from build123d import *

# Parameters (mm, degrees)
F0_W        = 127
F0_H        = 127
F1_DEPTH    = 19.05
F2_T1_DEPTH = 257.6414957887
F2_T3_DEPTH = 257.6414957887
F3_T        = -2.54
F4_W        = 63.5
F4_H        = 63.5
F5_DEPTH    = 25.4


# Not quite as in the source:
# - a fillet or chamfer that OpenCascade refuses, or shapes differently, is made with other operations: its cross-section is extruded or revolved along the edge and cut away or added


with BuildPart() as f1:
    # F0 (on Front) → F1 (new body)
    with BuildSketch(Plane.XZ):
        with Locations((-51.5997745097, 45.6864875067)):
            Rectangle(F0_W, F0_H)
    extrude(amount=F1_DEPTH)

    # F2: chamfer of 25.4 on 4 edges, made by hand

    # F2_s2 → F2_t1 (cut)
    with BuildSketch(Plane.XY.offset(-83.1342603876)):
        Polygon((11.9002254903, 6.35), (-13.4997745097, -19.05), (11.9002254903, -19.05), align=None)
        Polygon((-115.0997745097, 6.35), (-89.6997745097, -19.05), (-115.0997745097, -19.05), align=None)
    extrude(amount=F2_T1_DEPTH, mode=Mode.SUBTRACT)

    # F2_s4 → F2_t3 (cut)
    with BuildSketch(Plane.YZ.offset(-180.420522404)):
        Polygon((6.35, 109.1864875067), (-19.05, 83.7864875067), (-19.05, 109.1864875067), align=None)
        Polygon((6.35, -17.8135124933), (-19.05, 7.5864875067), (-19.05, -17.8135124933), align=None)
    extrude(amount=F2_T3_DEPTH, mode=Mode.SUBTRACT)

    # F3
    f3_openings = [f1.faces().sort_by_distance(p)[0] for p in [
        (-51.599775, -19.05, 45.686488),
    ]]
    offset(amount=F3_T, openings=f3_openings, kind=Kind.INTERSECTION)

    # F4 (on face) → F5 (cut)
    with BuildSketch(Plane(origin=(0, 0, 0), x_dir=(-1, 0, 0), z_dir=(0, 1, 0))):
        with Locations((51.5997745097, 45.6864875067)):
            Rectangle(F4_W, F4_H)
    extrude(amount=-F5_DEPTH, mode=Mode.SUBTRACT)


solid = f1.part
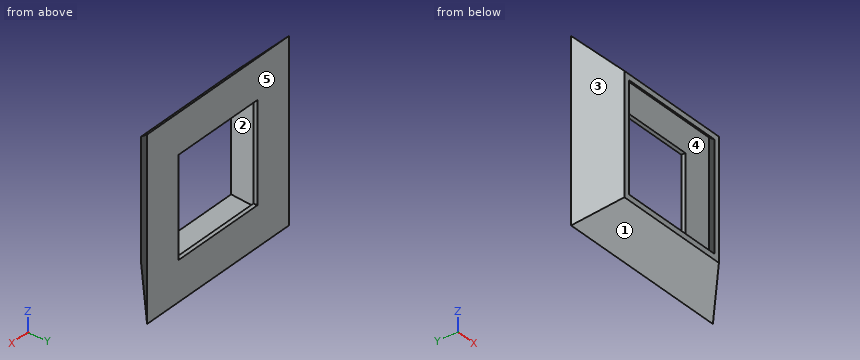
Build history of the part. All positions in model axes, mm. Face numbers are marked on the shaded views. A direction names the side the tool comes from. Coordinates: 2 decimals unless noted, no trailing zeros. Write each loop counter-clockwise with the first axis right and the second up, starting at its lowest first coordinate (ties: lowest second). Pieces come first, ordered by that corner, then holes. Notation, with made-up numbers: (60.5, 14) -> (115.5, 14) arc R33 ccw to (115.5, 48) -> close; hole circle Ø9 at (-17, -25.75). An arc over 180 degrees is marked (long way). Use CSV: the item, a comma, the result in double quotes. Start each with the question number.
Q1. Pull direction Y, two halves, no side cores. Call the marked faces 3, 4 and 5: released by +Y, released by -Y, zero draft, split by the parting line, or undercut.
Q2. Cut at B-B, the plane z = 18. List the corners of the cut face in (x, y), then the cut area to 3 significant figures.
Q3. Flat gauge pins, fed straight in: pin 1 Ø12 at (x, z) = (-83.5, 39.5) entering from -Y; pin 2 Ø1.5 at (x, y) = (-82.5, -12.5) entering from +Z; pin 3 Ø5 at (x, y) = (-52, -14) entering from -Z; pin 4 Ø3 at (x, y) = (-32.5, -10.5) entering from -Z. Where does each tip first touch, or does it go through?
Q4. Cut at C-C, the plane y = -5.75. List the corners of the cut face in (x, z).
Q5. Cut at A-A, the plane x = -57. List the corners of the cut face in (y, z).
Q6. 3-axis set-ups, long thin cutter, end or side, ignore diameter. For the marked faces 1 and 2: which of +Z, -Z, +X, -X, +Y, -Y reach the whole face in a straight line?
Q7. Drill centre lines: probe 1 along Z at (x, y) = (-32, -14.75); probe 2 along Z at (x, y) = (-90.5, -14); probe 3 along Y at (x, z) = (-67, -3). Where is each one in solid material? Low to high.
Q8. Cut at D-D, the plane x = -92. List the corners of the cut face in (y, z), then the cut area to 3 significant figures.
Checked values:
1,face 3,"released by -Y"
1,face 4,"undercut"
1,face 5,"released by +Y"
2,outline,"(-108.75, 0) -> (-89.7, -19.05) -> (-86.11, -19.05) -> (-102.62, -2.54) -> (-83.35, -2.54) -> (-83.35, 0) -> close; (-19.85, -2.54) -> (-0.58, -2.54) -> (-17.09, -19.05) -> (-13.5, -19.05) -> (5.55, 0) -> (-19.85, 0) -> close"
2,area,"241 mm²"
3,pin 1,"stops at y = -19.05"
3,pin 2,"stops at z = 91.09"
3,pin 3,"stops at z = 0.04"
3,pin 4,"stops at z = -2.46"
4,outline,"(-103, -5.71) -> (-0.2, -5.71) -> (-0.2, 97.09) -> (-103, 97.09) -> close; hole (-99.41, -2.12) -> (-3.79, -2.12) -> (-3.79, 93.49) -> (-99.41, 93.49) -> close"
5,outline,"(-19.05, 7.59) -> (0, -11.46) -> (0, 13.94) -> (-2.54, 13.94) -> (-2.54, -5.33) -> (-19.05, 11.18) -> close; (-19.05, 80.19) -> (-2.54, 96.7) -> (-2.54, 77.44) -> (0, 77.44) -> (0, 102.84) -> (-19.05, 83.79) -> close"
6,face 1,"-Z, +X, -X, -Y"
6,face 2,"none"
7,probe 1,"z = 3.29 to 6.88, 84.49 to 88.09"
7,probe 2,"z = 2.54 to 6.13, 85.24 to 88.84"
7,probe 3,"y = -8.46 to -4.87, -2.54 to 0"
8,outline,"(-16.75, 5.29) -> (0, -11.46) -> (0, 102.84) -> (-16.75, 86.09) -> close; hole (-13.16, 5.29) -> (-2.54, -5.33) -> (-2.54, 96.7) -> (-13.16, 86.09) -> close"
8,area,"663 mm²"
